```python
from build123d import *

# Parameters (mm, degrees)
BOSS_EXTRUDE1_DEPTH = 2


with BuildPart() as part:
    # Sketch1 → Boss-Extrude1 (new body)
    with BuildSketch(Plane.XY):
        with BuildLine():
            Line((-10.396049823, -5.488799617), (-23.967764137, -5.488799617))
            ThreePointArc((-23.967764137, -5.488799617), (-21.24471958, -7.357273277), (-20.196049823, -10.488799617))
            ThreePointArc((-20.196049823, -10.488799617), (-21.24471958, -13.620325957), (-23.967764137, -15.488799617))
            Line((-23.967764137, -15.488799617), (-10.396049823, -15.488799617))
            Line((-10.396049823, -15.488799617), (-10.396049823, -5.488799617))
        make_face()
    extrude(amount=BOSS_EXTRUDE1_DEPTH)


solid = part.part
```
Can you work these out from the model? Positions are in its coordinate system, mm. Give positions to 0.01 mm unless a question says otherwise; leave off trailing zeros. Order: outer loops, then holes, each group sorted by start corner. A loop starts at its lowest first (then second) coordinate and runs counter-clockwise, first axis right, second up. Notation, with made-up numbers: M -29.5,11 L 20.5,11 A16 cw 20.5,25 Z; hole C -9.5,24.25 d1. An arc over 180 degrees is marked long. One line per item, written item: value.
1) I want a section at D-D, the plane y = -9.5. List the corners of the cut face in (x, z) for me.
Answer sheet:
outline: M -20.29,0 L -10.4,0 L -10.4,2 L -20.29,2 Z
2) I want a section at B-B, the plane x = -22.25. List the corners of the cut face in (y, z) for me.
Answer sheet:
outline: M -15.49,0 L -14.63,0 L -14.63,2 L -15.49,2 Z; M -6.35,0 L -5.49,0 L -5.49,2 L -6.35,2 Z
3) Please list where these lines run through material, in increasing order: line 1 along X through (y, z) = (-10.5, 1.55); line 2 along Y through (x, z) = (-22.5, 1.8); line 3 along Y through (x, z) = (-21.5, 1.25).
Answer sheet:
line 1: x = -20.2 to -10.4
line 2: y = -15.49 to -14.81, -6.17 to -5.49
line 3: y = -15.49 to -13.93, -7.04 to -5.49
4) For P1, Ø1, axis at y = -11.5, z = 0.5, coming from the -X side, with a flat end and sliding along its axis, tell me the tip position at first contact or that it passes through.
Answer sheet:
P1: stops at x = -20.42
5) I want a section at A-A, the plane z = 1.7. List the corners of the cut face in (x, y) for me, plus the area to 3 significant figures.
Answer sheet:
outline: M -23.97,-15.49 L -10.4,-15.49 L -10.4,-5.49 L -23.97,-5.49 A5.2 cw Z
area: 108 mm^2
6) I want a section at C-C, the plane y = -11. List the corners of the cut face in (x, z) for me.
Answer sheet:
outline: M -20.22,0 L -10.4,0 L -10.4,2 L -20.22,2 Z
